The model under review builds one solid part; all positions refer to its coordinate system, in mm. A direction names the side the tool comes from. Coordinates: 2 decimals unless noted, no trailing zeros. Loops run counter-clockwise (first coordinate to the right, second up) from the corner with the lowest first, then second, coordinate; pieces in that order, holes last. Notation, with made-up numbers: (-24.75, 64.5) - (-6.75, 64.5) arc R21 ccw to (-6.75, 82.5) - close; hole circle Ø8 at (-18.5, 57). An arc over 180 degrees is marked (long way). Use a Markdown table: item, result. Add a question column.
1) Add section D-D, the plane x = 4. Give the boundary of the cut face in (y, z).
2) Clearance check with flat-ended pins moving along their axes: pin 1 (1 mm diameter, centred on y = 2, z = -42, fed in from -X); pin 2 (2 mm diameter, centred on x = -3, z = -24, fed in from -Y); pin 3 (1.5 mm diameter, centred on x = -2.5, z = -47.5, fed in from +Y). State where each tip first meets the part, or that it passes through.
3) To check wall thickness, follow L1, parallel to X at y = 0.75, z = -27.5; L2, parallel to Z at x = 1, y = 2; L3, parallel to Y at x = -4, z = 1.5. State the ranges of each line that lie inside material, in increasing order. Write a range as [from, to].
4) For faces 1 (the flat face through (6.5, 0, 0)), 2 (the cylindrical face through (2.8, 0.1, -47.2)), list the 3-axis set-ups (+Z, -Z, +X, -X, +Y, -Y) from which the entire face can be reached by the end or side of a thin tool; tool diameter is ignored.
5) Add section C-C, the plane z = -54.5. Give the boundary of the cut face in (x, y).
```python
from build123d import *

# Parameters (mm, degrees)
SKETCH1_R               = 4.5
BOSS_EXTRUDE1_DEPTH     = 6.5
SKETCH2_R               = 3
BOSS_EXTRUDE2_DEPTH     = 60
CUT_EXTRUDE_THIN1_START = -25
SKETCH3_R               = 3
SKETCH3_R_2             = 2.8
CUT_EXTRUDE_THIN1_DEPTH = 25
CHAMFER1_SIZE2          = 0.2
CHAMFER1_SIZE           = 0.549495484
CHAMFER2_SIZE           = 0.2
CHAMFER3_SIZE           = 0.2


with BuildPart() as part:
    # Sketch1 → Boss-Extrude1 (new, symmetric)
    with BuildSketch(Plane(origin=(0, 0, 0), x_dir=(0, 0, -1), z_dir=(1, 0, 0))):
        with Locations(Location((0, 0, 0), (0, 0, 180))):
            Circle(SKETCH1_R)
    extrude(amount=BOSS_EXTRUDE1_DEPTH, both=True)

    # Sketch2 → Boss-Extrude2 (add)
    with BuildSketch(Plane.XY):
        Circle(SKETCH2_R)
    extrude(amount=-BOSS_EXTRUDE2_DEPTH)

    # Sketch3 → Cut-Extrude-Thin1 (cut)
    with BuildSketch(Plane(origin=(0, 0, -60), x_dir=(-1, 0, 0), z_dir=(0, 0, -1)).offset(CUT_EXTRUDE_THIN1_START)):
        Circle(SKETCH3_R)
        Circle(SKETCH3_R_2, mode=Mode.SUBTRACT)
    extrude(amount=CUT_EXTRUDE_THIN1_DEPTH, mode=Mode.SUBTRACT)

    # Chamfer1
    chamfer1_edges = [part.edges().sort_by_distance(p)[0] for p in [
        (-3, 0, -35),
    ]]
    chamfer1_side = [part.faces().sort_by_distance(p)[0] for p in [
        (-3, 0, -34.996),
    ]]
    chamfer(chamfer1_edges, length=CHAMFER1_SIZE - 0.0001, length2=CHAMFER1_SIZE2 - 0.0001, reference=chamfer1_side[0])  # a hair under: the kernel refuses the full size

    # Chamfer2
    chamfer2_edges = [part.edges().sort_by_distance(p)[0] for p in [
        (-6.5, 0, -4.5),
        (6.5, 0, -4.5),
    ]]
    chamfer(chamfer2_edges, length=CHAMFER2_SIZE)

    # Chamfer3
    chamfer3_edges = [part.edges().sort_by_distance(p)[0] for p in [
        (2.8, 0, -60),
    ]]
    chamfer(chamfer3_edges, length=CHAMFER3_SIZE)


solid = part.part
```
From the geometry:
| question | item | result |
|---|---|---|
| 1 | outline | circle Ø9 at (0, 0) |
| 2 | pin 1 | stops at x = -2.36 |
| 2 | pin 2 | stops at y = -2.24 |
| 2 | pin 3 | stops at y = 2.19 |
| 3 | L1 | x = [-2.9, 2.9] |
| 3 | L2 | z = [-60, 4.03] |
| 3 | L3 | y = [-4.24, 4.24] |
| 4 | face 1 | +Z, -Z, +X, +Y, -Y |
| 4 | face 2 | -Z |
| 5 | outline | circle Ø5.6 at (0, 0) |
